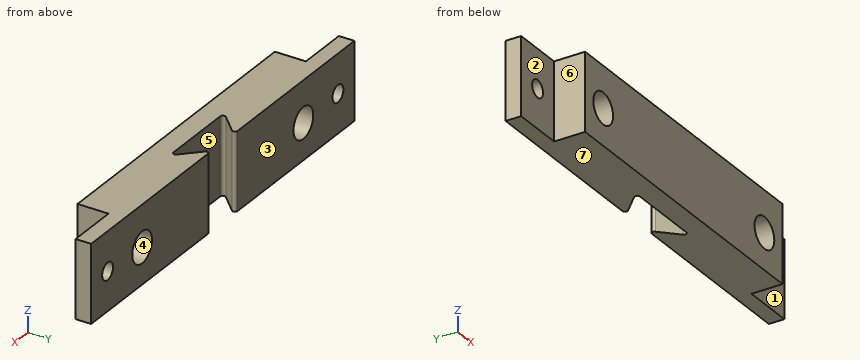
```python
from build123d import *

# Parameters (mm, degrees)
SKETCH_1_W               = 60
SKETCH_1_H               = 15
SKETCH_1_R               = 3
EXTRUDE_1_DEPTH          = 6
EXTRUDE_START            = 6
SKETCH_1_3_W             = 80
SKETCH_1_3_H             = 15
SKETCH_1_3_R             = 1.65
SKETCH_1_3_R_2           = 3
EXTRUDE_2_DEPTH          = 3
CUT_EXTRUDE_1_DEPTH      = 42.680331093
CUT_EXTRUDE_1_DEPTH_BACK = 42.680331093


with BuildPart() as part:
    # Эскиз1 → Бобышка-Вытянуть1 (new body)
    with BuildSketch(Plane(origin=(0, 0, 0), x_dir=(1, 0, 0), z_dir=(0, 1, 0))):
        Rectangle(SKETCH_1_W, SKETCH_1_H)
        with Locations(Location((24.5, 0.5, 0), (0, 0, 270))):
            Circle(SKETCH_1_R, mode=Mode.SUBTRACT)
        with Locations(Location((-24.5, 0.5, 0), (0, 0, 270))):
            Circle(SKETCH_1_R, mode=Mode.SUBTRACT)
    extrude(amount=EXTRUDE_1_DEPTH)

    # Эскиз1<3> → Бобышка-Вытянуть2 (add)
    with BuildSketch(Plane(origin=(0, 0, 0), x_dir=(1, 0, 0), z_dir=(0, 1, 0)).offset(EXTRUDE_START)):
        Rectangle(SKETCH_1_3_W, SKETCH_1_3_H)
        with Locations(Location((-35, 0, 0), (0, 0, 270))):
            Circle(SKETCH_1_3_R, mode=Mode.SUBTRACT)
        with Locations(Location((24.5, 0.5, 0), (0, 0, 270))):
            Circle(SKETCH_1_3_R_2, mode=Mode.SUBTRACT)
        with Locations(Location((-24.5, 0.5, 0), (0, 0, 270))):
            Circle(SKETCH_1_3_R_2, mode=Mode.SUBTRACT)
        with Locations(Location((35, 0, 0), (0, 0, 270))):
            Circle(SKETCH_1_3_R, mode=Mode.SUBTRACT)
    extrude(amount=EXTRUDE_2_DEPTH)

    # Эскиз2 → Вырез-Вытянуть1 (cut, two sides: drawn at the far end of the back side and taken through both)
    with BuildSketch(Plane.XY.offset(-CUT_EXTRUDE_1_DEPTH_BACK)):
        with BuildLine():
            Line((4.153553391, 8.146446609), (7.446446609, 4.853553391))
            ThreePointArc((7.446446609, 4.853553391), (7.554832985, 4.308658284), (7.092893219, 4))
            Line((7.092893219, 4), (-7.092893219, 4))
            ThreePointArc((-7.092893219, 4), (-7.554832985, 4.308658284), (-7.446446609, 4.853553391))
            Line((-7.446446609, 4.853553391), (-4.153553391, 8.146446609))
            ThreePointArc((-4.153553391, 8.146446609), (-4.045167015, 8.691341716), (-4.507106781, 9))
            Line((-4.507106781, 9), (4.507106781, 9))
            ThreePointArc((4.507106781, 9), (4.045167015, 8.691341716), (4.153553391, 8.146446609))
        make_face()
    extrude(amount=CUT_EXTRUDE_1_DEPTH + CUT_EXTRUDE_1_DEPTH_BACK, mode=Mode.SUBTRACT)


solid = part.part
```
Geometry: final body of the model. Coordinates: model frame, mm. Face numbers are marked on the shaded views. A direction names the side the tool comes from. Coordinates: 2 decimals unless noted, no trailing zeros. Loops run counter-clockwise (first coordinate to the right, second up) from the corner with the lowest first, then second, coordinate; pieces in that order, holes last. Notation, with made-up numbers: M 60.25,19 L 70.25,19 A19 cw 70.25,41 Z; hole C 10.5,-39.75 d8. An arc over 180 degrees is marked long. Put each result on its own line as item: value.
(1) Cut plane B-B on x = -35. Return the cut outline in (y, z).
Answer sheet:
outline: M 6,-7.5 L 9,-7.5 L 9,-1.65 L 6,-1.65 Z; M 6,1.65 L 9,1.65 L 9,7.5 L 6,7.5 Z
(2) Cut plane D-D on y = 1.75. Return the cut outline in (x, z), then the cut area to 3 significant figures.
Answer sheet:
outline: M -30,-7.5 L 30,-7.5 L 30,7.5 L -30,7.5 Z; hole C -24.5,-0.5 d6; hole C 24.5,-0.5 d6
area: 843 mm^2
(3) First-contact query: pin 1 (5.5 mm diameter, centred on x = -35, z = 0, fed in from -Y); pin 2 (2 mm diameter, centred on y = 4.5, z = 0.5, fed in from +X); pin 3 (2 mm diameter, centred on x = -11.5, z = 2.5, fed in from -Y); pin 4 (4.5 mm diameter, centred on x = 1.5, z = -2.5, fed in from +Y). Flat tips, straight axial feed; report the tip coordinate or a pass-through.
Answer sheet:
pin 1: stops at y = 6
pin 2: stops at x = 30
pin 3: stops at y = 0
pin 4: stops at y = 4
(4) Access query for the marked faces 1, 2 and 3. Directions: +Z, -Z, +X, -X, +Y, -Y. A direction counts if a zero-diameter tool reaches every point of the face in a straight line with its end or side. Return the directions, or none.
Answer sheet:
face 1: +Z, -Z, +X, -Y
face 2: +Z, -Z, -X, -Y
face 3: +Z, -Z, +X, -X, +Y
(5) Cut plane C-C on z = 0. State how many separate pieces and enclosed holes the cut face has, then the cut area to 3 significant figures.
Answer sheet:
separate pieces: 5
enclosed holes: 0
area: 416 mm^2
(6) Draft query along X for the marked faces 4, 5, 6 and 7. Return one class per face: pulls with the +X half, pulls with the -X half, needs draft (parallel to the pull), parting line crosses it, or undercut.
Answer sheet:
face 4: undercut
face 5: undercut
face 6: pulls with the -X half
face 7: needs draft
(7) Material intervals for probe 1 along X at (y, z) = (8, 2); probe 2 along X at (y, z) = (7.25, 1.5); probe 3 along X at (y, z) = (8.15, 0), sorted ascending.
Answer sheet:
probe 1: x = -40 to -26.16, -22.84 to -4.3, 4.3 to 22.84, 26.16 to 40
probe 2: x = -40 to -35.69, -34.31 to -26.74, -22.26 to -5.05, 5.05 to 22.26, 26.74 to 34.31, 35.69 to 40
probe 3: x = -40 to -36.65, -33.35 to -27.46, -21.54 to -4.15, 4.15 to 21.54, 27.46 to 33.35, 36.65 to 40
(8) Cut plane A-A on y = 7.25. Return the cut outline in (x, z).
Answer sheet:
outline: M -40,-7.5 L -5.05,-7.5 L -5.05,7.5 L -40,7.5 Z; M 5.05,-7.5 L 40,-7.5 L 40,7.5 L 5.05,7.5 Z; hole C -35,0 d3.3; hole C -24.5,-0.5 d6; hole C 24.5,-0.5 d6; hole C 35,0 d3.3
